```python
from build123d import *

# Parameters (mm, degrees)
SKETCH1_3_W         = 80
SKETCH1_3_H         = 80
SKETCH1_3_R         = 15
SKETCH1_3_R_2       = 2.5
BOSS_EXTRUDE3_DEPTH = 5
BOSS_EXTRUDE4_START = 5
SKETCH1_W           = 80
SKETCH1_H           = 80
SKETCH1_R           = 2.5
SKETCH1_R_2         = 25
BOSS_EXTRUDE4_DEPTH = 5
CUT_EXTRUDE1_DEPTH  = 90.582364336


with BuildPart() as part:
    # Sketch1_3 → Boss-Extrude3 (new body)
    with BuildSketch(Plane(origin=(0, 0, 0), x_dir=(1, 0, 0), z_dir=(0, 1, 0))):
        Rectangle(SKETCH1_3_W, SKETCH1_3_H)
        with Locations(Location((0, 0, 0), (0, 0, 270))):
            Circle(SKETCH1_3_R, mode=Mode.SUBTRACT)
        with Locations(Location((-32, 32, 0), (0, 0, 270))):
            Circle(SKETCH1_3_R_2, mode=Mode.SUBTRACT)
        with Locations(Location((-32, -32, 0), (0, 0, 270))):
            Circle(SKETCH1_3_R_2, mode=Mode.SUBTRACT)
        with Locations(Location((32, -32, 0), (0, 0, 270))):
            Circle(SKETCH1_3_R_2, mode=Mode.SUBTRACT)
        with Locations(Location((32, 32, 0), (0, 0, 270))):
            Circle(SKETCH1_3_R_2, mode=Mode.SUBTRACT)
    extrude(amount=-BOSS_EXTRUDE3_DEPTH)

    # Sketch1 → Boss-Extrude4 (add)
    with BuildSketch(Plane(origin=(0, 0, 0), x_dir=(1, 0, 0), z_dir=(0, 1, 0)).offset(BOSS_EXTRUDE4_START)):
        Rectangle(SKETCH1_W, SKETCH1_H)
        with Locations(Location((-32, -32, 0), (0, 0, 270))):
            Circle(SKETCH1_R, mode=Mode.SUBTRACT)
        with Locations(Location((32, -32, 0), (0, 0, 270))):
            Circle(SKETCH1_R, mode=Mode.SUBTRACT)
        with Locations(Location((0, 0, 0), (0, 0, 270))):
            Circle(SKETCH1_R_2, mode=Mode.SUBTRACT)
        with Locations(Location((-32, 32, 0), (0, 0, 270))):
            Circle(SKETCH1_R, mode=Mode.SUBTRACT)
        with Locations(Location((32, 32, 0), (0, 0, 270))):
            Circle(SKETCH1_R, mode=Mode.SUBTRACT)
    extrude(amount=-BOSS_EXTRUDE4_DEPTH)

    # Sketch5 → Cut-Extrude1 (cut, through all)
    with BuildSketch(Plane(origin=(0, 0, -40), x_dir=(-1, 0, 0), z_dir=(0, 0, -1))):
        with BuildLine():
            Line((40, 5), (-40, 5))
            ThreePointArc((-40, 5), (0, 2.128129211), (40, 5))
        make_face()
    extrude(amount=-CUT_EXTRUDE1_DEPTH, mode=Mode.SUBTRACT)


solid = part.part
```
Here's how the part is built. I have some questions about the finished solid (model axes, mm). A direction names the side the tool comes from. Coordinates: 2 decimals unless noted, no trailing zeros. Loops run counter-clockwise (first coordinate to the right, second up) from the corner with the lowest first, then second, coordinate; pieces in that order, holes last. Notation, with made-up numbers: (42.25, 70.5) -> (69.25, 70.5) arc R11 ccw to (69.25, 88.5) -> close; hole circle Ø3 at (50.25, 87.25). An arc over 180 degrees is marked (long way). Return JSON: item names as keys, results as strings.
1) If we section it at A-A, the plane z = 0: Write out the boundary of the cut face in (x, y), then the cut area to 3 significant figures.
Results below:
{"outline": "(-40, -5) -> (-15, -5) -> (-15, 0) -> (-25, 0) -> (-25, 3.25) arc R280 cw to (-40, 5) -> close; (15, -5) -> (40, -5) -> (40, 5) arc R280 cw to (25, 3.25) -> (25, 0) -> (15, 0) -> close", "area": "372 mm²"}
2) Will these pins go through, and if not, where does the flat tip stop? pin 1 (2 mm diameter, centred on x = -8, z = 18.5, fed in from +Y); pin 2 (4 mm diameter, centred on x = 32, z = 32, fed in from +Y); pin 3 (5 mm diameter, centred on x = -24.5, z = 13.5, fed in from +Y).
Results below:
{"pin 1": "y = 0", "pin 2": "through", "pin 3": "y = 3.43"}
3) If we section it at D-D, the plane x = 5.5: Write out the boundary of the cut face in (y, z).
Results below:
{"outline": "(-5, -40) -> (2.18, -40) -> (2.18, -24.39) -> (0, -24.39) -> (0, -13.96) -> (-5, -13.96) -> close; (-5, 13.96) -> (0, 13.96) -> (0, 24.39) -> (2.18, 24.39) -> (2.18, 40) -> (-5, 40) -> close"}
4) For faces 1 (the face through (-1, -1, -40)), 2 (the face through (11, 0, 11)), which set-ups out of +Z, -Z, +X, -X, +Y, -Y let a thin tool reach every point of the face, with its end or its side?
Results below:
{"face 1": "-Z, +X, -X, +Y, -Y", "face 2": "+Y"}
5) Thinking about a two-plate mould opening in X: for faces 3 (the face through (40, 0, 1)), 4 (the face through (17, -5, -1)), 5 (the face through (-40, 0, 1)), 6 (the face through (1.099, 1.286, -24.976)), which applies, +X half, -X half, draft (parallel to the pull), parting line (faces both ways), or undercut?
Results below:
{"face 3": "+X half", "face 4": "draft", "face 5": "-X half", "face 6": "undercut"}
6) I need wall thicknesses on line 1 (X direction, y = -0.75, z = -32); line 2 (Z direction, x = -31.5, y = 2). Which ranges of each line are inside material? Lowest first, please. Write a range as from..to.
Results below:
{"line 1": "-40..-34.5, -29.5..29.5, 34.5..40", "line 2": "-40..-34.45, -29.55..29.55, 34.45..40"}
7) If we section it at B-B, the plane y = -3.5: Write out the boundary of the cut face in (x, z).
Results below:
{"outline": "(-40, -40) -> (40, -40) -> (40, 40) -> (-40, 40) -> close; hole circle Ø5 at (-32, -32); hole circle Ø5 at (-32, 32); hole circle Ø30 at (0, 0); hole circle Ø5 at (32, -32); hole circle Ø5 at (32, 32)"}
8) If we section it at C-C, the plane x = 31: Write out the boundary of the cut face in (y, z).
Results below:
{"outline": "(-5, -40) -> (3.85, -40) -> (3.85, -34.29) -> (-5, -34.29) -> close; (-5, -29.71) -> (3.85, -29.71) -> (3.85, 29.71) -> (-5, 29.71) -> close; (-5, 34.29) -> (3.85, 34.29) -> (3.85, 40) -> (-5, 40) -> close"}
